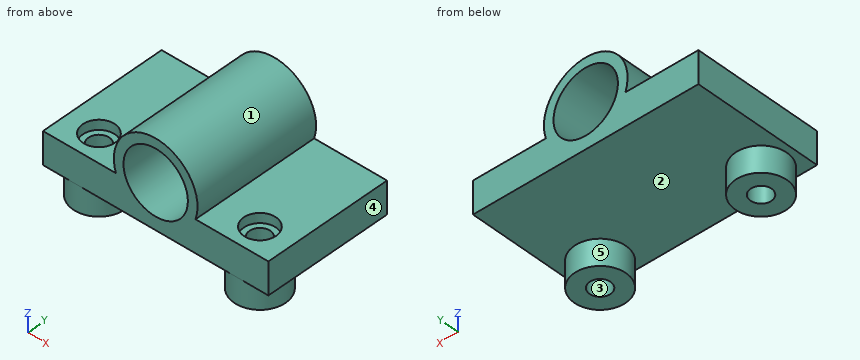
from build123d import *

# Parameters (mm, degrees)
SKETCH002_AS_DRAWN_R                 = 13
SKETCH002_AS_DRAWN_R_2               = 10
EXTRUDE002_DEPTH                     = 40
EXTRUDE002_ONTO_SKETCH002_ROLL_ANGLE = 90
SKETCH003_AS_DRAWN_R                 = 13
EXTRUDE003_DEPTH                     = 40
EXTRUDE003_ONTO_SKETCH003_ROLL_ANGLE = 90
SKETCH_W                             = 70
SKETCH_H                             = 40
SKETCH_R                             = 5
EXTRUDE_DEPTH                        = 10
SKETCH001_R                          = 8
SKETCH001_R_2                        = 3.25
EXTRUDE001_DEPTH                     = 15


with BuildPart() as extrude002:
    # Sketch002 as drawn → Extrude002 (new)
    with BuildSketch(Plane.XY):
        Circle(SKETCH002_AS_DRAWN_R)
        Circle(SKETCH002_AS_DRAWN_R_2, mode=Mode.SUBTRACT)
    extrude(amount=-EXTRUDE002_DEPTH)


with BuildPart() as extrude002_1:
    # Extrude002 onto Sketch002 roll: moved
    add(extrude002.part.rotate(Axis((0, 0, 0), (1, 0, 0)), EXTRUDE002_ONTO_SKETCH002_ROLL_ANGLE))


with BuildPart() as extrude002_2:
    # Extrude002 onto Sketch002 placement: moved
    add(extrude002_1.part)


with BuildPart() as extrude002_3:
    # Extrude002 placement: moved
    add(extrude002_2.part.moved(Location((0, -20, 14))))


with BuildPart() as extrude003:
    # Sketch003 as drawn → Extrude003 (new)
    with BuildSketch(Plane.XY):
        Circle(SKETCH003_AS_DRAWN_R)
    extrude(amount=-EXTRUDE003_DEPTH)


with BuildPart() as extrude003_1:
    # Extrude003 onto Sketch003 roll: moved
    add(extrude003.part.rotate(Axis((0, 0, 0), (1, 0, 0)), EXTRUDE003_ONTO_SKETCH003_ROLL_ANGLE))


with BuildPart() as extrude003_2:
    # Extrude003 onto Sketch003 placement: moved
    add(extrude003_1.part)


with BuildPart() as extrude003_3:
    # Extrude003 placement: moved
    add(extrude003_2.part.moved(Location((0, -20, 14))))


with BuildPart() as cut:
    # Sketch → Extrude (new body)
    with BuildSketch(Plane.XY):
        Rectangle(SKETCH_W, SKETCH_H)
        with Locations((-25, -12)):
            Circle(SKETCH_R, mode=Mode.SUBTRACT)
        with Locations((25, -12)):
            Circle(SKETCH_R, mode=Mode.SUBTRACT)
    extrude(amount=EXTRUDE_DEPTH)

    # Cut: cut Extrude003
    add(extrude003_3.part, mode=Mode.SUBTRACT)


with BuildPart() as fusion:
    # Sketch001 → Extrude001 (new body)
    with BuildSketch(Plane.XY):
        with Locations((-25, -12)):
            Circle(SKETCH001_R)
        with Locations((-25, -12)):
            Circle(SKETCH001_R_2, mode=Mode.SUBTRACT)
        with Locations((25, -12)):
            Circle(SKETCH001_R)
        with Locations((25, -12)):
            Circle(SKETCH001_R_2, mode=Mode.SUBTRACT)
    extrude(amount=EXTRUDE001_DEPTH)


with BuildPart() as fusion_1:
    # Extrude001 placement: moved
    add(fusion.part.moved(Location((0, 0, -8))))

    # Fusion: union Extrude002, Cut
    add(extrude002_3.part)
    add(cut.part)


solid = fusion_1.part
Verification items for the finished model (mm, model axes). Face numbers are marked on the shaded views. A direction names the side the tool comes from. Coordinates: 2 decimals unless noted, no trailing zeros. Write each loop counter-clockwise with the first axis right and the second up, starting at its lowest first coordinate (ties: lowest second). Pieces come first, ordered by that corner, then holes. Notation, with made-up numbers: M 34.5,67.25 L 44.5,67.25 A20 ccw 44.5,100.25 Z; hole C 8.25,49.5 d10. An arc over 180 degrees is marked long. One line per question, with ' | ' between items.
1) Sectioned sample at B-B on x = 0. Record the cut outline in (y, z).
Solutions:
outline: M -20,0 L 20,0 L 20,4 L -20,4 Z; M -20,24 L 20,24 L 20,27 L -20,27 Z
2) Sectioned sample at C-C on z = 14. Record the cut outline in (x, y).
Solutions:
outline: M -13,-20 L -10,-20 L -10,20 L -13,20 Z; M 10,-20 L 13,-20 L 13,20 L 10,20 Z
3) Depth check by flat-ended pin: pin 1 Ø8 at (x, z) = (-18.5, 18) entering from -Y; pin 2 Ø1.5 at (y, z) = (-8.5, 17) entering from +X; pin 3 Ø8 at (x, y) = (23, -12) entering from +Z; pin 4 Ø5 at (y, z) = (7.5, 19) entering from -X. Enter the tip coordinate at first touch or a pass-through.
Solutions:
pin 1: through | pin 2: x = 12.8 | pin 3: z = 10 | pin 4: x = -12.76
4) Sectioned sample at D-D on y = 10. Record the cut outline in (x, z).
Solutions:
outline: M -35,0 L 35,0 L 35,10 L 12.37,10 A13 ccw long -12.37,10 L -35,10 Z; hole C 0,14 d20
5) Material ranges on L1, parallel to Y at x = -25, z = 8.35; L2, parallel to Z at x = 0, y = -11; L3, parallel to X at y = -12, z = 9.3, recorded low to high.
Solutions:
L1: -20 to -17, -7 to 20 | L2: 0 to 4, 24 to 27 | L3: -35 to -30, -20 to -8.83, 8.83 to 20, 30 to 35
6) Release check for a two-part mould opening along Z. For the marked faces 1, 2 and 3 record: +Z half, -Z half, draft (parallel to the pull), parting line (faces both ways), or undercut.
Solutions:
face 1: undercut | face 2: -Z half | face 3: draft
7) Sectioned sample at A-A on y = -12. State how many separate pieces and enclosed holes the cut face has, then the cut area to 3 significant figures.
Solutions:
separate pieces: 3 | enclosed holes: 1 | area: 755 mm^2
8) Access from +Z, -Z, +X, -X, +Y, -Y to the whole of each face (thin tool, end or side, straight path). Record for the marked faces 4 and 5.
Solutions:
face 4: +Z, -Z, +X, +Y, -Y | face 5: -Z
